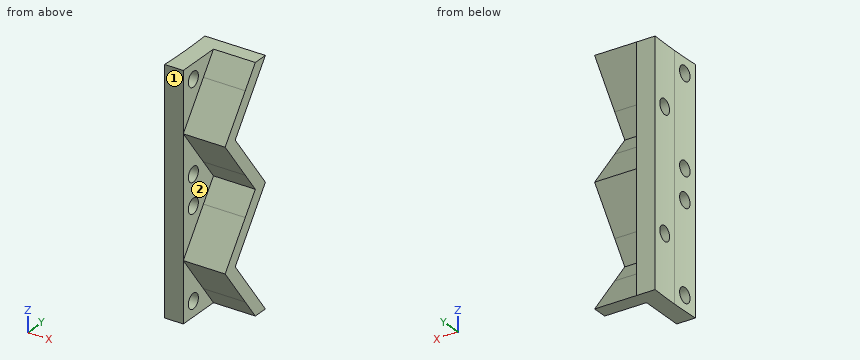
from build123d import *

# Parameters (mm, degrees)
SKETCH1_R           = 127
BOSS_EXTRUDE1_DEPTH = 50.8
SKETCH2_R           = 1.5875
BOSS_EXTRUDE2_DEPTH = 15.24
SKETCH2_4_R         = 1.5875
CUT_EXTRUDE1_DEPTH  = 8.89
LPATTERN1_COUNT     = 2
LPATTERN1_PITCH     = 25.4
SKETCH1_2_R         = 127
CUT_EXTRUDE2_DEPTH  = 51.8


with BuildPart() as part:
    # Sketch1 → Boss-Extrude1 (new body)
    with BuildSketch(Plane.XY):
        Circle(SKETCH1_R)
    extrude(amount=BOSS_EXTRUDE1_DEPTH)


with BuildPart() as body_2:
    # Sketch2 → Boss-Extrude2 (new body)
    with BuildSketch(Plane(origin=(139.7, 0, 0), x_dir=(0, 0, -1), z_dir=(1, 0, 0))):
        Polygon((0, -6.35), (0, 0), (-4.233333333, 0), (-12.7, -6.35), align=None)
        with Locations((-3.175, -3.175)):
            Circle(SKETCH2_R, mode=Mode.SUBTRACT)
        Polygon((-4.233333333, 0), (0, 0), (0, 3.175), align=None)
        Polygon((-16.933333333, 0), (-8.466666667, 0), (0, 6.35), (-25.4, 6.35), align=None)
        with Locations((-12.7, 3.175)):
            Circle(SKETCH2_R, mode=Mode.SUBTRACT)
        Polygon((-12.7, -3.175), (-8.466666667, 0), (-16.933333333, 0), align=None)
        Polygon((-25.4, -6.35), (-12.7, -6.35), (-21.166666667, 0), (-25.4, 0), align=None)
        with Locations((-22.225, -3.175)):
            Circle(SKETCH2_R, mode=Mode.SUBTRACT)
        Polygon((-25.4, 0), (-21.166666667, 0), (-25.4, 3.175), align=None)
        Polygon((-12.7, -6.35), (-4.233333333, 0), (-8.466666667, 0), (-12.7, -3.175), (-16.933333333, 0), (-21.166666667, 0), align=None)
        Polygon((-21.166666667, 0), (-16.933333333, 0), (-25.4, 6.35), (-25.4, 3.175), align=None)
        Polygon((-8.466666667, 0), (-4.233333333, 0), (0, 3.175), (0, 6.35), align=None)
    extrude(amount=-BOSS_EXTRUDE2_DEPTH)

    # Sketch2_4 → Cut-Extrude1 (cut)
    with BuildSketch(Plane(origin=(139.7, 0, 0), x_dir=(0, 0, -1), z_dir=(1, 0, 0))):
        Polygon((0, -6.35), (0, 0), (-4.233333333, 0), (-12.7, -6.35), align=None)
        with Locations((-3.175, -3.175)):
            Circle(SKETCH2_4_R, mode=Mode.SUBTRACT)
        Polygon((-4.233333333, 0), (0, 0), (0, 3.175), align=None)
        Polygon((-16.933333333, 0), (-8.466666667, 0), (0, 6.35), (-25.4, 6.35), align=None)
        with Locations((-12.7, 3.175)):
            Circle(SKETCH2_4_R, mode=Mode.SUBTRACT)
        Polygon((-25.4, 0), (-21.166666667, 0), (-25.4, 3.175), align=None)
        Polygon((-12.7, -3.175), (-8.466666667, 0), (-16.933333333, 0), align=None)
        Polygon((-25.4, -6.35), (-12.7, -6.35), (-21.166666667, 0), (-25.4, 0), align=None)
        with Locations((-22.225, -3.175)):
            Circle(SKETCH2_4_R, mode=Mode.SUBTRACT)
    extrude(amount=-CUT_EXTRUDE1_DEPTH, mode=Mode.SUBTRACT)


with BuildPart() as lpattern1_1:
    # LPattern1: pattern copy
    add(body_2.part.moved(Location(Vector(0, 0, 1) * (1 * LPATTERN1_PITCH))))

    # Combine1: union body 2
    add(body_2.part)


with BuildPart() as cut_extrude2_tool:
    # Sketch1_2 → Cut-Extrude2 (new body, through all)
    with BuildSketch(Plane.XY):
        Circle(SKETCH1_2_R)
    extrude(amount=CUT_EXTRUDE2_DEPTH)


with BuildPart() as part_1:
    add(part.part)

    # Cut-Extrude2: cut by cut_extrude2_tool
    add(cut_extrude2_tool.part, mode=Mode.SUBTRACT)


with BuildPart() as lpattern1_1_1:
    add(lpattern1_1.part)

    # Cut-Extrude2: cut by cut_extrude2_tool
    add(cut_extrude2_tool.part, mode=Mode.SUBTRACT)


solid = lpattern1_1_1.part
Design review of the part built by this model. Coordinates are the model's own, in mm. Face numbers are marked on the shaded views. A direction names the side the tool comes from. Coordinates: 2 decimals unless noted, no trailing zeros. Write each loop counter-clockwise with the first axis right and the second up, starting at its lowest first coordinate (ties: lowest second). Pieces come first, ordered by that corner, then holes. Notation, with made-up numbers: (8, 63) - (48, 63) arc R19 cw to (48, 87) - close; hole circle Ø3 at (89.25, 39). An arc over 180 degrees is marked (long way). Use one line per item in the form item = value.
Q1. Consider section A-A (z = 37). Write out the cut boundary in (x, y) (3 decimals), plus the area to 3 significant figures.
Taken from the geometry:
outline = (126.841, -6.35) - (130.81, -6.35) - (130.81, -5.525) - (139.7, -5.525) - (139.7, -2.35) - (130.81, -2.35) - (130.81, 2.03) - (126.984, 2.03) arc R127 cw to start; (126.841, 6.35) arc R127 cw to (126.927, 4.32) - (130.81, 4.32) - (130.81, 6.35) - close
area = 68.5 mm^2
Q2. Consider section C-C (y = 3.75). Write out the cut boundary in (x, z).
Taken from the geometry:
outline = (126.94, 0) - (139.7, 0) - (139.7, 3.47) - (130.81, 3.47) - (130.81, 11.22) - (126.94, 11.22) - close; (126.94, 14.18) - (130.81, 14.18) - (130.81, 21.93) - (139.7, 21.93) - (139.7, 28.87) - (130.81, 28.87) - (130.81, 36.62) - (126.94, 36.62) - close; (126.94, 39.58) - (130.81, 39.58) - (130.81, 47.33) - (139.7, 47.33) - (139.7, 50.8) - (126.94, 50.8) - close
Q3. Machinability: for the marked faces 1 and 2, which of the approach directions +Z, -Z, +X, -X, +Y, -Y give a long, thin tool a straight path to every point of the face, cutting with its end or side? Answer none if there is none.
Taken from the geometry:
face_1 = +Z, -Z, +X, -X, -Y
face_2 = +X, -Y
Q4. Consider section D-D (y = 0.75). Write out the cut boundary in (x, z).
Taken from the geometry:
outline = (127, 0) - (130.81, 0) - (130.81, 3.23) - (139.7, 3.23) - (139.7, 7.47) - (130.81, 7.47) - (130.81, 17.93) - (139.7, 17.93) - (139.7, 22.17) - (130.81, 22.17) - (130.81, 28.63) - (139.7, 28.63) - (139.7, 32.87) - (130.81, 32.87) - (130.81, 43.33) - (139.7, 43.33) - (139.7, 47.57) - (130.81, 47.57) - (130.81, 50.8) - (127, 50.8) - close
Q5. Consider section B-B (x = 130). Count the separate pieces of the cut face and the enclosed holes in it, plus the area to 3 significant figures.
Taken from the geometry:
separate_pieces = 1
enclosed_holes = 6
area = 598 mm^2
Q6. Insertion check: pin 1 Ø4 at (y, z) = (-3.175, 22.225) entering from +X; pin 2 Ø2 at (y, z) = (-3.5, 25) entering from -X; pin 3 Ø3 at (y, z) = (-3.175, 47.625) entering from -X; pin 4 Ø2 at (x, z) = (132.5, 5.5) entering from -Y. Each pin has a flat end and moves straight along its axis. Give the tip position at first contact, or say it passes through.
Taken from the geometry:
pin_1 = 130.81
pin_2 = 126.92
pin_3 = through
pin_4 = -1.7
Q7. For probe 1 along Y at (x, z) = (128.65, 38.1); probe 2 along Z at (x, y) = (130.5, -2.5); probe 3 along Z at (x, y) = (137.75, 4.5), list the stretches that pass through material, from the lowest coordinate up.
Taken from the geometry:
probe_1 = -6.35 to 1.59, 4.76 to 6.35
probe_2 = 0 to 1.74, 4.61 to 20.79, 23.66 to 27.14, 30.01 to 46.19, 49.06 to 50.8
probe_3 = 0 to 2.47, 22.93 to 27.87, 48.33 to 50.8
